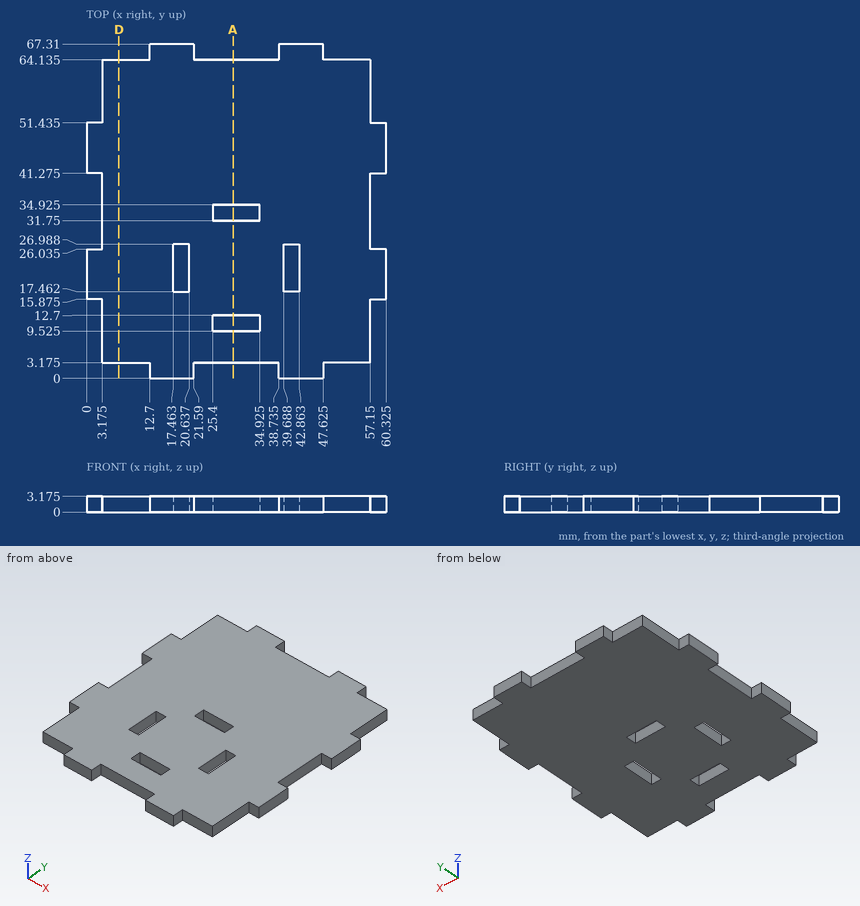
Check sheet for the drawn part. Datum: minimum x, y, z corner. Units: mm. Coordinates: 2 decimals unless noted, no trailing zeros. Order: outer loops, then holes, each group sorted by start corner. A loop starts at its lowest first (then second) coordinate and runs counter-clockwise, first axis right, second up. Notation, with made-up numbers: M -34.5,-10 L 0.5,-10 A18 ccw 0.5,3 Z; hole C 58.25,38 d4. An arc over 180 degrees is marked long. One line per item, written item: value. Start each with the question number.
Item 1: Scan lines: probe 1 along X at (y, z) = (25.5, 1.3) (1 decimal); probe 2 along Y at (x, z) = (20.5, 0.75); probe 3 along Y at (x, z) = (11, 0.95) (1 decimal). Record each from-to range of solid material in increasing order.
Item 2: Gauge pin test, flat ends, axial feed: pin 1 (1.6 mm diameter, centred on y = 22, z = 2, fed in from -X); pin 2 (1 mm diameter, centred on x = 10, z = 1, fed in from +Y) (1 decimal); pin 3 (1.5 mm diameter, centred on x = 36, z = 1.5, fed in from -Y) (1 decimal); pin 4 (1 mm diameter, centred on y = 8, z = 1, fed in from +X). Record the tip position at first contact, or that the pin passes through.
Item 3: Sectioned sample at A-A (x = 29.5). Count the separate pieces of the cut face and the enclosed holes in it.
Item 4: Sectioned sample at D-D (x = 6.5). Enter the section's corners in (y, z) (1 decimal).
Conclusion:
1. probe 1: x = 0 to 17.5, 20.6 to 39.7, 42.9 to 60.3
1. probe 2: y = 0 to 17.46, 26.99 to 67.31
1. probe 3: y = 3.2 to 64.1
2. pin 1: stops at x = 0
2. pin 2: stops at y = 64.1
2. pin 3: stops at y = 3.2
2. pin 4: stops at x = 57.15
3. separate pieces: 3
3. enclosed holes: 0
4. outline: M 3.2,0 L 64.1,0 L 64.1,3.2 L 3.2,3.2 Z
